```python
from build123d import *

# Parameters (mm, degrees)
F1_DEPTH = 28.575
F0_W     = 25.4
F0_H     = 25.4
F0_R     = 1.984375
F2_DEPTH = 3.175
F3_R     = 1.984375
F5_DEPTH = 25.4
F4_R     = 1.984375
F6_DEPTH = 25.4


with BuildPart() as f1:
    # F0 (on Top) → F1 (new body)
    with BuildSketch(Plane.XY):
        Polygon((-11.1125, 12.7), (-14.2875, 12.7), (-14.2875, -12.7), (-14.2875, -15.875), (14.2875, -15.875), (14.2875, -12.7), (-11.1125, -12.7), align=None)
    extrude(amount=F1_DEPTH)

    # F0 (on Top) → F2 (join)
    with BuildSketch(Plane.XY):
        with Locations((1.5875, 0)):
            Rectangle(F0_W, F0_H)
        with Locations((-4.7625, -6.35)):
            Circle(F0_R, mode=Mode.SUBTRACT)
        with Locations((7.9375, -6.35)):
            Circle(F0_R, mode=Mode.SUBTRACT)
        with Locations((-4.7625, 6.35)):
            Circle(F0_R, mode=Mode.SUBTRACT)
        with Locations((7.9375, 6.35)):
            Circle(F0_R, mode=Mode.SUBTRACT)
    extrude(amount=F2_DEPTH)

    # F3 (on face) → F5 (cut)
    with BuildSketch(Plane(origin=(-14.2875, 0, 0), x_dir=(0, -1, 0), z_dir=(-1, 0, 0))):
        with Locations((-6.35, 22.225)):
            Circle(F3_R)
        with Locations((6.35, 22.225)):
            Circle(F3_R)
        with Locations((6.35, 9.525)):
            Circle(F3_R)
        with Locations((-6.35, 9.525)):
            Circle(F3_R)
    extrude(amount=-F5_DEPTH, mode=Mode.SUBTRACT)

    # F4 (on face) → F6 (cut)
    with BuildSketch(Plane.XZ.offset(15.875)):
        with Locations((7.9375, 22.225)):
            Circle(F4_R)
        with Locations((7.9375, 9.525)):
            Circle(F4_R)
        with Locations((-4.7625, 9.525)):
            Circle(F4_R)
        with Locations((-4.7625, 22.225)):
            Circle(F4_R)
    extrude(amount=-F6_DEPTH, mode=Mode.SUBTRACT)


solid = f1.part
```
The model under review builds one solid part; all positions refer to its coordinate system, in mm. A direction names the side the tool comes from. Give positions to 0.01 mm unless a question says otherwise; leave off trailing zeros. Write each loop counter-clockwise with the first axis right and the second up, starting at its lowest first coordinate (ties: lowest second). Pieces come first, ordered by that corner, then holes. Notation, with made-up numbers: M 28.25,3.25 L 33.25,3.25 A23 ccw 33.25,13.25 Z; hole C 82,39.5 d2. An arc over 180 degrees is marked long. Answer in a Markdown table with one row per item.
Item 1: For line 1 along Y through (x, z) = (-1.25, 9.5) (3 decimals); line 2 along Z through (x, y) = (12.25, -9.75) (3 decimals); line 3 along X through (y, z) = (2.5, 11.5), list the stretches that pass through material, from the lowest coordinate up.
Check sheet entries:
| item | result |
|---|---|
| line 1 | -15.875 to -12.7 |
| line 2 | 0 to 3.175 |
| line 3 | -14.29 to -11.11 |
Item 2: Draft analysis for pull direction Z (two halves, no side actions). For faces 1 (the face through (7.679, -14.31, 24.192)), 2 (the face through (14.288, -13, 8)), 3 (the face through (1, 0, 3.175)), 4 (the face through (-5.021, -14.31, 11.492)), state which applies: +Z half, -Z half, draft (parallel to the pull), parting line (faces both ways), or undercut.
Check sheet entries:
| item | result |
|---|---|
| face 1 | undercut |
| face 2 | draft |
| face 3 | +Z half |
| face 4 | undercut |
Item 3: Add section A-A on y = 6.35. Give the boundary of the cut face in (x, z) (1 decimal), plus the area to 3 significant figures.
Check sheet entries:
| item | result |
|---|---|
| outline | M -14.3,0 L -6.7,0 L -6.7,3.2 L -11.1,3.2 L -11.1,7.5 L -14.3,7.5 Z; M -14.3,11.5 L -11.1,11.5 L -11.1,20.2 L -14.3,20.2 Z; M -14.3,24.2 L -11.1,24.2 L -11.1,28.6 L -14.3,28.6 Z; M -2.8,0 L 6,0 L 6,3.2 L -2.8,3.2 Z; M 9.9,0 L 14.3,0 L 14.3,3.2 L 9.9,3.2 Z |
| area | 121 mm2 |
Item 4: For P1, Ø5, axis at y = -6.35, z = 9.525, coming from the +X side; P2, Ø6.5, axis at x = -4.76, z = 9.52, coming from the +Y side; P3, Ø3, axis at x = 10, y = -5.5, coming from the +Z side (3 decimals); P4, Ø2.5, axis at x = 7.94, y = -6.35, coming from the +Z side, all flat-tipped, find the tip position at first contact; note any pin that passes through.
Check sheet entries:
| item | result |
|---|---|
| P1 | x = -11.11 |
| P2 | y = -12.7 |
| P3 | z = 3.175 |
| P4 | through |
Item 5: Add section B-B on x = 8.75. Give the boundary of the cut face in (y, z) (3 decimals).
Check sheet entries:
| item | result |
|---|---|
| outline | M -15.875,0 L -8.16,0 L -8.16,3.175 L -12.7,3.175 L -12.7,7.715 L -15.875,7.715 Z; M -15.875,11.335 L -12.7,11.335 L -12.7,20.415 L -15.875,20.415 Z; M -15.875,24.035 L -12.7,24.035 L -12.7,28.575 L -15.875,28.575 Z; M -4.54,0 L 4.54,0 L 4.54,3.175 L -4.54,3.175 Z; M 8.16,0 L 12.7,0 L 12.7,3.175 L 8.16,3.175 Z |
Item 6: Add section C-C on z = 2.75. State how many separate pieces and enclosed holes the cut face has, plus the area to 3 significant figures.
Check sheet entries:
| item | result |
|---|---|
| separate pieces | 1 |
| enclosed holes | 4 |
| area | 767 mm2 |
Item 7: Add section D-D on x = -9. Give the boundary of the cut face in (y, z) (3 decimals), plus the area to 3 significant figures.
Check sheet entries:
| item | result |
|---|---|
| outline | M -15.875,0 L 12.7,0 L 12.7,3.175 L -12.7,3.175 L -12.7,28.575 L -15.875,28.575 Z |
| area | 171 mm2 |
Item 8: Tool access review of faces 5 (the face through (2, -12.7, 16)), 6 (the face through (-12.72, -4.89, 10.87)): name each direction out of +Z, -Z, +X, -X, +Y, -Y from which nothing blocks a thin tool from reaching the whole face with its end or side.
Check sheet entries:
| item | result |
|---|---|
| face 5 | +Z, +X, +Y |
| face 6 | +X, -X |
